Autodesk Inventor part; units mm, degrees
ref_plane "YZ Plane" through (0, 0, 0) normal (1, 0, 0) x (0, 1, 0)
ref_plane "XZ Plane" through (0, 0, 0) normal (0, 1, 0) x (-1, 0, 0)
ref_plane "XY Plane" through (0, 0, 0) normal (0, 0, 1) x (1, 0, 0)
sketch "Sketch1" plane through (0, 0, 0) normal (0, 0, 1) x (1, 0, 0)
  line L0 (12.5, -12) -> (-12.5, -12)
  line L1 (-12.5, -12) -> (-12.5, 12)
  line L2 (-12.5, 12) -> (12.5, 12)
  line L3 (12.5, 12) -> (12.5, -12)
  line L4 (12.5, -12) -> (-12.5, 12) construction
  line L5 (-12.5, -12) -> (12.5, 12) construction
  point P0 (0, 0)
  dimension "d0" = 24
  dimension "d1" = 25
extrude "Extrusion1" add sketch "Sketch1" along normal mid plane 1
sketch "Sketch2" plane through (0, 0, -0.5) normal (0, 0, -1) x (-1, 0, 0)
  line L0 (-5.5, 3.5) -> (5.5, 3.5)
  line L1 (5.5, 3.5) -> (5.5, -7.5)
  line L2 (5.5, -7.5) -> (-5.5, -7.5)
  line L3 (-5.5, -7.5) -> (-5.5, 3.5)
  line L4 (-5.5, 3.5) -> (5.5, -7.5) construction
  line L5 (5.5, 3.5) -> (-5.5, -7.5) construction
  line L6 (-12.5, -12) -> (12.5, -12)
  point P0 (0, 0)
  point P1 (0, -2)
  point P2 (0, -2)
  dimension "d4" = 11
  dimension "d5" = 11
  dimension "d6" = 4.5
extrude "Extrusion2" add sketch "Sketch2" along normal blind 5
sketch "Sketch3" plane through (0, 0, -0.5) normal (0, 0, -1) x (-1, 0, 0)
  circle A0 centre (0, -2) radius 4.5
  line L0 (5.5, 3.5) -> (-5.5, 3.5)
  line L1 (5.5, -7.5) -> (5.5, 3.5)
  point P0 (0, 0)
  point P1 (0, 3.5)
  point P2 (5.5, -2)
  dimension "d9" = 9
extrude "Extrusion3" add sketch "Sketch3" along normal blind 8
sketch "Sketch4" plane through (0, 0, -0.5) normal (0, 0, -1) x (-1, 0, 0)
  line L0 (3, 6) -> (-5.5, 6)
  line L1 (-5.5, 6) -> (-5.5, 10)
  line L2 (-5.5, 10) -> (3, 10)
  line L3 (3, 10) -> (3, 6)
  line L4 (3, 6) -> (-5.5, 10) construction
  line L5 (-5.5, 6) -> (3, 10) construction
  line L6 (12.5, 12) -> (-12.5, 12)
  line L7 (-12.5, 12) -> (-12.5, -12)
  point P0 (0, 0)
  point P1 (-1.25, 8)
  dimension "d12" = 8.5
  dimension "d13" = 4
  dimension "d14" = 2
  dimension "d15" = 7
extrude "Extrusion4" add sketch "Sketch4" along normal blind 1.5
sketch "Sketch5" plane through (0, 0, -0.5) normal (0, 0, -1) x (-1, 0, 0)
  line L0 (11.5, -4) -> (-11.5, -4) construction
  line L1 (-11.5, -4) -> (-11.5, 11) construction
  line L2 (-11.5, 11) -> (11.5, 11) construction
  line L3 (11.5, 11) -> (11.5, -4) construction
  line L4 (11.5, -4) -> (-11.5, 11) construction
  line L5 (-11.5, -4) -> (11.5, 11) construction
  line L6 (12.5, 12) -> (-12.5, 12)
  line L7 (12.5, -12) -> (12.5, 12)
  circle A0 centre (-10.5, 10) radius 1
  circle A1 centre (10.5, 10) radius 1
  circle A2 centre (-10.5, -3) radius 1
  circle A3 centre (10.5, -3) radius 1
  point P0 (0, 0)
  point P1 (0, 3.5)
  point P2 (0, 11)
  point P3 (0, 12)
  dimension "d19" = 15
  dimension "d20" = 1
  dimension "d21" = 1
  dimension "d22" = 2
  dimension "d23" = 2
  dimension "d24" = 2
  dimension "d25" = 2
extrude "Extrusion5" cut sketch "Sketch5" against normal through all
sketch "Sketch6" plane through (0, 0, -0.5) normal (0, 0, 1) x (1, 0, 0)
  line L0 (-10.5, -12) -> (10.5, -12)
  line L1 (10.5, -12) -> (10.5, -6)
  line L2 (10.5, -6) -> (-10.5, -6)
  line L3 (-10.5, -6) -> (-10.5, -12)
  line L4 (-10.5, -12) -> (10.5, -6) construction
  line L5 (10.5, -12) -> (-10.5, -6) construction
  line L6 (-12.5, -12) -> (12.5, -12)
  point P0 (0, 0)
  point P1 (0, -9)
  point P2 (0, -9)
  dimension "d28" = 21
  dimension "d29" = 6
extrude "Extrusion6" add sketch "Sketch6" along normal blind 4
fillet "Fillet1" radius 2 4 edges at (12.5, 12, 0) (12.5, -12, 0) (-12.5, 12, 0) (-12.5, -12, 0)
equation "\"d5\" = d4"
equation "\"d23\" = d22"
equation "\"d24\" = d22"
equation "\"d25\" = d24"
properties part number "raspberry pi camera v2"
For this review, take the finished solid that the model builds, in its own axes (mm). A direction names the side the tool comes from. Coordinates: 2 decimals unless noted, no trailing zeros. Loops run counter-clockwise (first coordinate to the right, second up) from the corner with the lowest first, then second, coordinate; pieces in that order, holes last. Notation, with made-up numbers: (77.25, -5) -> (119.25, -5) arc R25 cw to (119.25, 29) -> close; hole circle Ø10 at (37, -11). An arc over 180 degrees is marked (long way). Write each question's results on one line, items separated by ' | '.
Q1. Machinability: for faces 5 (the flat face through (-5.5, -2, -3)), 6 (the flat face through (10.5, -9, 2)), 7 (the flat face through (0, -7.5, -3)), which of the approach directions +Z, -Z, +X, -X, +Y, -Y give a long, thin tool a straight path to every point of the face, cutting with its end or side? Answer none if there is none.
Taken from the geometry:
face 5: -Z, -X, +Y, -Y | face 6: +Z, +X, +Y, -Y | face 7: -Z, +X, -X, -Y
Q2. For pin 1 Ø12 at (x, y) = (-9.5, -4) entering from +Z; pin 2 Ø1 at (x, z) = (-2, -3) entering from +Y; pin 3 Ø1 at (x, y) = (-7, 0.5) entering from -Z; pin 4 Ø0.9 at (x, z) = (3.5, 2.5) entering from +Y, all flat-tipped, find the tip position at first contact; note any pin that passes through.
Taken from the geometry:
pin 1: z = 3.5 | pin 2: y = 3.5 | pin 3: z = -0.5 | pin 4: y = -6
Q3. Add section A-A, the plane x = -5. State the section outline as (y, z) points, then the cut area to 3 significant figures.
Taken from the geometry:
outline: (-12, -0.5) -> (-7.5, -0.5) -> (-7.5, -5.5) -> (3.5, -5.5) -> (3.5, -0.5) -> (12, -0.5) -> (12, 0.5) -> (-6, 0.5) -> (-6, 3.5) -> (-12, 3.5) -> close | area: 97.0 mm²
Q4. Mouldability with a two-part tool opening along Y and no side actions: class faces 1 (the flat face through (0, 3.5, -3)), 2 (the flat face through (-12.5, 0, 0)), 3 (the cylindrical face through (-11.93, 11.4, -0.01)), 4 (the cylindrical face through (-9.7, -3.6, 0)) as +Y half, -Y half, draft (parallel to the pull), parting line (faces both ways), or undercut.
Taken from the geometry:
face 1: undercut | face 2: draft | face 3: +Y half | face 4: undercut
Q5. Add section D-D, the plane z = -3.5. State the section outline as (x, y) points, then the cut area to 3 significant figures.
Taken from the geometry:
outline: (-5.5, -7.5) -> (5.5, -7.5) -> (5.5, 3.5) -> (-5.5, 3.5) -> close | area: 121 mm²
Q6. Add section C-C, the plane x = 11. State the section outline as (y, z) points.
Taken from the geometry:
outline: (-11.94, -0.5) -> (-3.87, -0.5) -> (-3.87, 0.5) -> (-11.94, 0.5) -> close; (-2.13, -0.5) -> (9.13, -0.5) -> (9.13, 0.5) -> (-2.13, 0.5) -> close; (10.87, -0.5) -> (11.94, -0.5) -> (11.94, 0.5) -> (10.87, 0.5) -> close
Q7. Add section B-B, the plane y = -3.5. State the section outline as (x, z) points.
Taken from the geometry:
outline: (-12.5, -0.5) -> (-11.37, -0.5) -> (-11.37, 0.5) -> (-12.5, 0.5) -> close; (-9.63, -0.5) -> (-5.5, -0.5) -> (-5.5, -5.5) -> (-4.24, -5.5) -> (-4.24, -8.5) -> (4.24, -8.5) -> (4.24, -5.5) -> (5.5, -5.5) -> (5.5, -0.5) -> (9.63, -0.5) -> (9.63, 0.5) -> (-9.63, 0.5) -> close; (11.37, -0.5) -> (12.5, -0.5) -> (12.5, 0.5) -> (11.37, 0.5) -> close
Q8. To check wall thickness, follow line 1 along Y through (x, z) = (-10.5, -0.05); line 2 along Z through (x, y) = (-3.75, 0.75); line 3 along Z through (x, y) = (-1.75, -11). State the ranges of each line that lie inside material, in increasing order. Write a range as [from, to].
Taken from the geometry:
line 1: [-12, -4], [-2, 9], [11, 12] | line 2: [-5.5, 0.5] | line 3: [-0.5, 3.5]
